Design review of the part built by this model. Coordinates are the model's own, in mm. A direction names the side the tool comes from. Coordinates: 2 decimals unless noted, no trailing zeros. Loops run counter-clockwise (first coordinate to the right, second up) from the corner with the lowest first, then second, coordinate; pieces in that order, holes last. Notation, with made-up numbers: (12, 55) -> (67, 55) arc R24 cw to (67, 66) -> close; hole circle Ø4 at (58.25, 27.5). An arc over 180 degrees is marked (long way). Use CSV: the item, a comma, the result in double quotes.
```python
from build123d import *

# Parameters (mm, degrees)
BOSS_EXTRUDE1_DEPTH      = 10
BOSS_EXTRUDE2_DEPTH      = 10
BOSS_EXTRUDE3_DEPTH      = 10
BOSS_EXTRUDE3_DEPTH_BACK = 50
SKETCH3_R                = 7.5


with BuildPart() as part:
    # Sketch1 → Boss-Extrude1 (new body)
    with BuildSketch(Plane(origin=(0, 0, 0), x_dir=(1, 0, 0), z_dir=(0, 1, 0))):
        with BuildLine():
            Line((-107.529653027, 53.267004046), (-89.608044189, 44.389170038))
            ThreePointArc((-89.608044189, 44.389170038), (-0.97130255, 99.995282746), (88.728870826, 46.121442756))
            Line((88.728870826, 46.121442756), (106.474644991, 55.345731307))
            ThreePointArc((106.474644991, 55.345731307), (-1.16556306, 119.994339295), (-107.529653027, 53.267004046))
        make_face()
    extrude(amount=BOSS_EXTRUDE1_DEPTH)

    # Sketch2 → Boss-Extrude2 (add)
    with BuildSketch(Plane(origin=(0, 10, 0), x_dir=(1, 0, 0), z_dir=(0, 1, 0))):
        with BuildLine():
            Line((-62.097280291, 96.793221769), (-56.697516787, 88.376419876))
            ThreePointArc((-56.697516787, 88.376419876), (0, 105), (56.697516787, 88.376419876))
            Line((56.697516787, 88.376419876), (62.097280291, 96.793221769))
            ThreePointArc((62.097280291, 96.793221769), (0, 115), (-62.097280291, 96.793221769))
        make_face()
    extrude(amount=BOSS_EXTRUDE2_DEPTH)

    # Mirror1: part across plane


with BuildPart() as part_1:
    add(part.part)
    add(part.part.mirror(Plane.ZX.offset(20)))

    # Sketch3 → Boss-Extrude3 (add, two sides: drawn at the far end of the back side and taken through both)
    with BuildSketch(Plane.XZ.offset(-BOSS_EXTRUDE3_DEPTH_BACK)):
        with Locations(Location((-89.658117345, -63.616209095, 0), (0, 0, 270))):
            Circle(SKETCH3_R)
    extrude(amount=BOSS_EXTRUDE3_DEPTH + BOSS_EXTRUDE3_DEPTH_BACK)

    # Mirror2: part across plane


with BuildPart() as part_2:
    add(part_1.part)
    add(part_1.part.mirror(Plane(origin=(0, 0, 0), x_dir=(0, 0, 1), z_dir=(1, 0, 0))))


solid = part_2.part
```
Item 1: Draft analysis for pull direction X (two halves, no side actions). For faces 1 (the face through (59.36, 20.14, -92.53)), 2 (the face through (-82.22, 20.14, -62.64)), 3 (the face through (90, -10, -64)), state which applies: pulls with the +X half, pulls with the -X half, needs draft (parallel to the pull), parting line crosses it, or undercut.
Checked values:
face 1,"pulls with the +X half"
face 2,"undercut"
face 3,"needs draft"
Item 2: To check wall thickness, follow line 1 along Y through (x, z) = (3, -104); line 2 along X through (y, z) = (37.5, -63); line 3 along Z through (x, y) = (2.5, 4.5). State the ranges of each line that lie inside material, in increasing order.
Checked values:
line 1,"0 to 10, 30 to 40"
line 2,"-102.13 to -77.66, 77.66 to 102.13"
line 3,"-119.97 to -99.97"
Item 3: Add section A-A (x = -67.5). Give the boundary of the cut face in (y, z).
Checked values:
outline,"(0, -99.22) -> (10, -99.22) -> (10, -73.78) -> (0, -73.78) -> close; (30, -99.22) -> (40, -99.22) -> (40, -73.78) -> (30, -73.78) -> close"
Item 4: Add section B-B (z = -80.5). Give the boundary of the cut face in (x, y), then the cut area to 3 significant figures.
Checked values:
outline,"(-88.99, 0) -> (-59.33, 0) -> (-59.33, 10) -> (-88.99, 10) -> close; (-88.99, 30) -> (-59.33, 30) -> (-59.33, 40) -> (-88.99, 40) -> close; (59.33, 0) -> (88.99, 0) -> (88.99, 10) -> (59.33, 10) -> close; (59.33, 30) -> (88.99, 30) -> (88.99, 40) -> (59.33, 40) -> close"
area,"1,190 mm^2"
Item 5: Add section D-D (x = 0.5). Give the boundary of the cut face in (y, z), then the cut area to 3 significant figures.
Checked values:
outline,"(0, -120) -> (10, -120) -> (10, -115) -> (30, -115) -> (30, -120) -> (40, -120) -> (40, -100) -> (30, -100) -> (30, -105) -> (10, -105) -> (10, -100) -> (0, -100) -> close"
area,"600 mm^2"
Item 6: Add section C-C (y = 19). Give the boundary of the cut face in (x, z), then the cut area to 3 significant figures.
Checked values:
outline,"circle Ø15 at (-89.66, -63.62); (-62.1, -96.79) arc R115 ccw to (62.1, -96.79) -> (56.7, -88.38) arc R105 cw to (-56.7, -88.38) -> close; circle Ø15 at (89.66, -63.62)"
area,"1,610 mm^2"
Item 7: Machinability: for faces 4 (the face through (82.22, -4.93, -62.64)), 5 (the face through (82.22, 45.07, -62.64)), 6 (the face through (-59.435, 20.14, -92.644)), 7 (the face through (-0.838, 20.14, -104.997)), which of the approach directions +Z, -Z, +X, -X, +Y, -Y give a long, thin tool a straight path to every point of the face, cutting with its end or side? Answer none if there is none.
Checked values:
face 4,"-Y"
face 5,"+Y"
face 6,"+Z, -X"
face 7,"+Z"
Item 8: Clearance check with flat-ended pins moving along their axes: pin 1 (10 mm diameter, centred on x = -54.5, y = -1, fed in from -Z); pin 2 (12 mm diameter, centred on x = -82.5, y = 15.5, fed in from -Z); pin 3 (1.5 mm diameter, centred on x = 80, y = 38.5, fed in from -Z). State where each tip first meets the part, or that it passes through.
Checked values:
pin 1,"z = -109.27"
pin 2,"z = -89.35"
pin 3,"z = -90.11"
